CAD build for the part. Positions are in the model's coordinates, mm. A direction names the side the tool comes from. Round coordinates to 2 decimals unless told otherwise and drop trailing zeros. Use one line per item in the form item = value.
from build123d import *

# Parameters (mm, degrees)
SKETCH1_R           = 4.15
BOSS_EXTRUDE1_DEPTH = 24
BOSS_EXTRUDE2_DEPTH = 12
SKETCH4_R           = 2.25
CUT_EXTRUDE1_DEPTH  = 51.135027226
CUT_EXTRUDE2_DEPTH  = 51.135027226
SKETCH6_R           = 10.9
CUT_EXTRUDE3_DEPTH  = 5
SKETCH7_R           = 4.5
CUT_EXTRUDE4_DEPTH  = 5
CUT_EXTRUDE5_REACH  = 58.104
SKETCH8_R           = 4.1
SKETCH10_R          = 3.25
CUT_EXTRUDE6_DEPTH  = 4
SKETCH11_R          = 1.75
CUT_EXTRUDE7_DEPTH  = 14


with BuildPart() as part:
    # Sketch1 → Boss-Extrude1 (new body)
    with BuildSketch(Plane.XY):
        with BuildLine():
            Line((13.341629993, -3.742589758), (7.682372306, -1.136974107))
            Line((7.682372306, -1.136974107), (-2.0678902, -23.426775412))
            Line((-2.0678902, -23.426775412), (-5.840324092, -21.776593778))
            ThreePointArc((-5.840324092, -21.776593778), (-7.962146661, -19.569683724), (-7.901980723, -16.508807532))
            Line((-7.901980723, -16.508807532), (-3.98023327, -7.54341081))
            add(Edge.make_bspline(
                [(-7.080436324, -0.68533899), (-4.531901983, -3.715550368), (-3.98023327, -7.54341081)],
                knots=[0, 0, 0, 1, 1, 1], degree=2))
            Line((-7.080436324, -0.68533899), (-29.803412918, 9.254408057))
            Line((-29.803412918, 9.254408057), (-27.798908258, 13.960167121))
            ThreePointArc((-27.798908258, 13.960167121), (-25.594658653, 16.110387521), (-22.515803889, 16.057307996))
            Line((-22.515803889, 16.057307996), (1.72881799, 5.451945282))
            add(Edge.make_bspline(
                [(1.72881799, 5.451945282), (9.747838199, 3.631364235), (13.341629993, -3.742589758)],
                knots=[0, 0, 0, 1, 1, 1], degree=2))
        make_face()
        Circle(SKETCH1_R, mode=Mode.SUBTRACT)
    extrude(amount=-BOSS_EXTRUDE1_DEPTH)

    # Sketch3 → Boss-Extrude2 (add)
    with BuildSketch(Plane(origin=(0, 0, -24), x_dir=(-1, 0, 0), z_dir=(0, 0, -1))):
        with BuildLine():
            Line((-7.682372306, -1.136974107), (-8.679331285, 2.212996201))
            add(Edge.make_bspline(
                [(-1.728818003, 5.451945279), (-5.764462803, 4.535721319), (-8.679331285, 2.212996201)],
                knots=[0, 0, 0, 1, 1, 1], degree=2))
            Line((-1.728818003, 5.451945279), (22.515803889, 16.057307996))
            ThreePointArc((22.515803889, 16.057307996), (25.594658653, 16.110387521), (27.798908258, 13.960167121))
            Line((27.798908258, 13.960167121), (28.304096394, 12.774191506))
            Line((28.304096394, 12.774191506), (3.510718988, 2.212996201))
            ThreePointArc((3.510718988, 2.212996201), (-3.681374953, -1.915718783), (3.826915418, 1.605371728))
            Line((3.826915418, 1.605371728), (28.62962492, 12.009983349))
            Line((28.62962492, 12.009983349), (29.803412918, 9.254408057))
            Line((29.803412918, 9.254408057), (7.080436358, -0.685338949))
            add(Edge.make_bspline(
                [(3.98023327, -7.54341081), (4.531901987, -3.715550342), (7.080436358, -0.685338949)],
                knots=[0, 0, 0, 1, 1, 1], degree=2))
            Line((3.98023327, -7.54341081), (-3.456922061, -10.796657252))
            Line((-3.456922061, -10.796657252), (-7.682372306, -1.136974107))
        make_face()
    extrude(amount=BOSS_EXTRUDE2_DEPTH)

    # Sketch4 → Cut-Extrude1 (cut, through all)
    with BuildSketch(Plane(origin=(-1.388852746, -3.17501726, 0), x_dir=(0.9161803596748023, -0.40076620185109174, 0), z_dir=(-0.4007662018510917, -0.9161803596748022, 0))):
        with Locations(Location((-13.70758094, -28.823038163, 0), (0, 0, 180))):
            Circle(SKETCH4_R)
    extrude(amount=-CUT_EXTRUDE1_DEPTH, mode=Mode.SUBTRACT)

    # Sketch5 → Cut-Extrude2 (cut, through all)
    with BuildSketch(Plane(origin=(-1.388852746, -3.17501726, 0), x_dir=(0.9161803596748023, -0.40076620185109174, 0), z_dir=(-0.4007662018510917, -0.9161803596748022, 0))):
        with BuildLine():
            Line((-18.149274911, -36), (-34.697304605, -37.023423696))
            Line((-34.697304605, -37.023423696), (-31.063763643, -18.422303423))
            add(Edge.make_bspline(
                [(-18.149274911, -36), (-21.35728774, -24.660432841), (-31.063763643, -18.422303423)],
                knots=[0, 0, 0, 1, 1, 1], degree=2))
        make_face()
    extrude(amount=-CUT_EXTRUDE2_DEPTH, mode=Mode.SUBTRACT)

    # Sketch6 → Cut-Extrude3 (cut)
    with BuildSketch(Plane(origin=(-1.388852746, -3.17501726, 0), x_dir=(0.9161803596748023, -0.40076620185109174, 0), z_dir=(-0.4007662018510917, -0.9161803596748022, 0))):
        with Locations((-17, -12.900000194)):
            Circle(SKETCH6_R)
    extrude(amount=-CUT_EXTRUDE3_DEPTH, mode=Mode.SUBTRACT)

    # Sketch7 → Cut-Extrude4 (cut)
    with BuildSketch(Plane(origin=(2.279484819, 5.211066233, 0), x_dir=(0.9161803596748023, -0.40076620185109163, 0), z_dir=(0.40076620185109163, 0.9161803596748023, 0))):
        with Locations(Location((-17, 12.900000194, 0), (0, 0, 180))):
            Circle(SKETCH7_R)
    extrude(amount=-CUT_EXTRUDE4_DEPTH, mode=Mode.SUBTRACT)

    # Cut-Extrude5: up to this plane
    cut_extrude5_end = Plane(origin=(13.341629993, -3.742589758, -24), z_dir=(-0.41821784159009956, -0.9083467603155299, 0))
    # Sketch8 → Cut-Extrude5 (cut, up to the surface)
    with BuildSketch(Plane(origin=(-8.933836899, -20.423393653, 0), x_dir=(0.9161803596748023, -0.4007662018510919, 0), z_dir=(-0.40076620185109185, -0.9161803596748022, 0)), mode=Mode.PRIVATE) as cut_extrude5_sk1:
        with Locations((9.5, -13.000000223)):
            Circle(SKETCH8_R)
    cut_extrude5_tool1 = split(extrude(cut_extrude5_sk1.sketch, amount=-CUT_EXTRUDE5_REACH, mode=Mode.PRIVATE), bisect_by=cut_extrude5_end, keep=Keep.BOTH, mode=Mode.PRIVATE)
    add(cut_extrude5_tool1.solids().sort_by_distance((-0.230123, -24.230673, -13))[0], mode=Mode.SUBTRACT)

    # Sketch10 → Cut-Extrude6 (cut)
    with BuildSketch(Plane(origin=(-0.571208632, 0.249864682, 0), x_dir=(0, 0, 1), z_dir=(-0.9161803596748025, 0.4007662018510913, 0))):
        with Locations(Location((-4.1353862, -13.399079912, 0), (0, 0, 270))):
            Circle(SKETCH10_R)
        with Locations(Location((-19.8646138, -13.399079912, 0), (0, 0, 270))):
            Circle(SKETCH10_R)
    extrude(amount=-CUT_EXTRUDE6_DEPTH, mode=Mode.SUBTRACT)

    # Sketch11 → Cut-Extrude7 (cut)
    with BuildSketch(Plane(origin=(3.093512806, -1.353200126, 0), x_dir=(0, 0, 1), z_dir=(-0.9161803596748025, 0.40076620185109135, 0))):
        with Locations(Location((-4.1353862, -13.399079912, 0), (0, 0, 270))):
            Circle(SKETCH11_R)
        with Locations(Location((-19.8646138, -13.399079912, 0), (0, 0, 270))):
            Circle(SKETCH11_R)
    extrude(amount=-CUT_EXTRUDE7_DEPTH, mode=Mode.SUBTRACT)


solid = part.part
1. Probe line 1 along Y through (x, z) = (0, -15.25); line 2 along Y through (x, z) = (0, -29); line 3 along Z through (x, y) = (10.5, -1.5). List the from-to ranges inside material, lowest first. Write a range as from..to.
Completed:
line_1 = -15.15..-4.15, 4.15..6.21
line_2 = -9.28..-4.15, 4.15..6.21
line_3 = -24..0
2. Cut at A-A on x = 0. State how many separate pieces and enclosed holes the cut face has, and give its area (3 significant figures).
Completed:
separate_pieces = 2
enclosed_holes = 2
area = 437 mm2
3. Pull direction Y, two halves, no side cores. Call faces 1 (the face through (-8, 1, 0)), 2 (the face through (-28.815, 11.574, -9.098)), 3 (the face through (2.875, -12.126, -4.646)), 4 (the face through (-0.265, -14.095, -21.573)): +Y half, -Y half, draft (parallel to the pull), parting line (faces both ways), or undercut.
Completed:
face_1 = draft
face_2 = +Y half
face_3 = -Y half
face_4 = undercut
4. Drop flat-ended pins along their axis: P1, Ø1, axis at x = 5, z = -17.5, coming from the -Y side; P2, Ø3, axis at x = 11, y = 0.5, coming from the -Z side; P3, Ø6, axis at y = 1, z = -7.5, coming from the +X side. Give the stop position or say it passes through.
Completed:
P1 = -8.41
P2 = -24
P3 = 12.38
5. Tool access for faces 5 (the face through (-11.01, 4.62, -31.25)), 6 (the face through (10, -1, -24)), 7 (the face through (-5, 1, -36)), 8 (the face through (-10.66, 6.34, -12.75)): list every direction of +Z, -Z, +X, -X, +Y, -Y with a clear straight run to the whole face (end or side of a thin tool).
Completed:
face_5 = -Z
face_6 = -Z, +X, -Y
face_7 = -Z, +X, -X, +Y, -Y
face_8 = none
